Read the model definition and answer for the solid it produces. Units are mm, in the model's axes. Face numbers are marked on the shaded views. A direction names the side the tool comes from. Give positions to 0.01 mm unless a question says otherwise; leave off trailing zeros. Write each loop counter-clockwise with the first axis right and the second up, starting at its lowest first coordinate (ties: lowest second). Pieces come first, ordered by that corner, then holes.
```python
from build123d import *

# Parameters (mm, degrees)
SKETCH1_W           = 28.956
SKETCH1_H           = 8.9916
SKETCH1_R           = 1.6002
BOSS_EXTRUDE1_DEPTH = 3.048
SKETCH2_W           = 7.62
SKETCH2_H           = 1.905
BOSS_EXTRUDE2_DEPTH = 6.35
FILLET1_R           = 0.254
FILLET2_R           = 0.635
CHAMFER1_SIZE       = 0.635


with BuildPart() as part:
    # Sketch1 → Boss-Extrude1 (new body)
    with BuildSketch(Plane(origin=(0, 0, 0), x_dir=(1, 0, 0), z_dir=(0, 1, 0))):
        Rectangle(SKETCH1_W, SKETCH1_H)
        with Locations(Location((8.128, 0, 0), (0, 0, 90))):
            Circle(SKETCH1_R, mode=Mode.SUBTRACT)
        with Locations(Location((-2.032, 0, 0), (0, 0, 90))):
            Circle(SKETCH1_R, mode=Mode.SUBTRACT)
    extrude(amount=BOSS_EXTRUDE1_DEPTH)

    # Sketch2 → Boss-Extrude2 (add)
    with BuildSketch(Plane.XY.offset(4.4958)):
        with Locations((-10.668, -0.9525)):
            Rectangle(SKETCH2_W, SKETCH2_H)
    extrude(amount=-BOSS_EXTRUDE2_DEPTH)

    # Fillet1
    fillet1_edges = [part.edges().sort_by_distance(p)[0] for p in [
        (-10.668, 0, -1.8542),
        (-6.858, 0, 1.3208),
    ]]
    fillet(fillet1_edges, radius=FILLET1_R)

    # Fillet2
    fillet2_edges = [part.edges().sort_by_distance(p)[0] for p in [
        (14.478, 1.524, 4.4958),
        (-14.478, 0.5715, 4.4958),
        (-14.478, 1.524, -4.4958),
        (14.478, 1.524, -4.4958),
    ]]
    fillet(fillet2_edges, radius=FILLET2_R)

    # Chamfer1
    chamfer1_edges = [part.edges().sort_by_distance(p)[0] for p in [
        (0, 3.048, -4.4958),
        (14.478, 3.048, 0),
        (-14.478, 3.048, 0),
        (0, 3.048, 4.4958),
        (-14.292012806, 3.048, -4.309812806),
        (-14.292012806, 3.048, 4.309812806),
        (14.292012806, 3.048, 4.309812806),
        (14.292012806, 3.048, -4.309812806),
    ]]
    chamfer(chamfer1_edges, length=CHAMFER1_SIZE)


solid = part.part
```
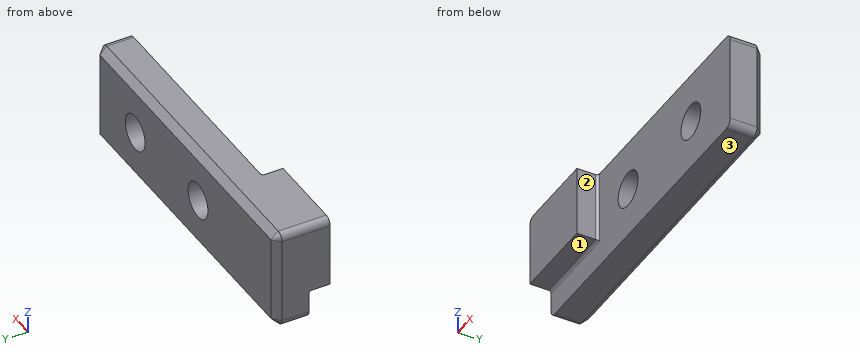
Item 1: Section A-A (z = 0) is taken. Write down the section's boundary in (x, y) (3 decimals).
Result set:
outline: (-14.478, -1.905) - (-6.858, -1.905) - (-6.858, -0.254) arc R0.254 cw to (-6.604, 0) - (-3.632, 0) - (-3.632, 3.048) - (-13.843, 3.048) - (-14.478, 2.413) - close; (-0.432, 0) - (6.528, 0) - (6.528, 3.048) - (-0.432, 3.048) - close; (9.728, 0) - (14.478, 0) - (14.478, 2.413) - (13.843, 3.048) - (9.728, 3.048) - close
Item 2: Find the intervals of material crossed by line 1 along X through (y, z) = (2.2, 0); line 2 along X through (y, z) = (2.55, 0.5); line 3 along X through (y, z) = (-0.4, -1), in increasing order.
Result set:
line 1: x = -14.48 to -3.63, -0.43 to 6.53, 9.73 to 14.48
line 2: x = -14.34 to -3.55, -0.51 to 6.61, 9.65 to 14.34
line 3: x = -14.48 to -6.86
Item 3: Each of these flat-tipped pins is pushed along its axis until it touches: pin 1 Ø3 at (x, z) = (8.128, 0) entering from +Y; pin 2 Ø4 at (x, z) = (-2.032, 0) entering from -Y; pin 3 Ø0.5 at (x, y) = (-11, -1) entering from -Z; pin 4 Ø1.3 at (y, z) = (-1.5, 0) entering from +X. Where does it stop, or does it pass through?
Result set:
pin 1: passes through
pin 2: stops at y = 0
pin 3: stops at z = -1.85
pin 4: stops at x = -6.86
Item 4: Section C-C (z = 2.5) is taken. Write down the section's boundary in (x, y) (3 decimals), and give its area (3 significant figures).
Result set:
outline: (-14.478, -1.905) - (-6.858, -1.905) - (-6.858, -0.254) arc R0.254 cw to (-6.604, 0) - (14.478, 0) - (14.478, 2.413) - (13.843, 3.048) - (-13.843, 3.048) - (-14.478, 2.413) - close
area: 102 mm2
Item 5: Section D-D (y = 1.65) is taken. Write down the section's boundary in (x, z) (3 decimals), and give its area (3 significant figures).
Result set:
outline: (-14.478, -3.861) arc R0.635 ccw to (-13.843, -4.496) - (13.843, -4.496) arc R0.635 ccw to (14.478, -3.861) - (14.478, 3.861) arc R0.635 ccw to (13.843, 4.496) - (-13.843, 4.496) arc R0.635 ccw to (-14.478, 3.861) - close; hole circle Ø3.2 at (-2.032, 0); hole circle Ø3.2 at (8.128, 0)
area: 244 mm2
Item 6: Which of the six approach directions +Z, -Z, +X, -X, +Y, -Y give full straight-line access (tool end or side, diameter ignored) to the marked faces 1, 2 and 3?
Result set:
face 1: -Z, +X, -X, -Y
face 2: +Z, -Z, +X, -Y
face 3: -Z, +X, -X, +Y, -Y
Item 7: Section B-B (x = 10.75) is taken. Write down the section's boundary in (y, z), and give its area (3 significant figures).
Result set:
outline: (0, -4.5) - (2.41, -4.5) - (3.05, -3.86) - (3.05, 3.86) - (2.41, 4.5) - (0, 4.5) - close
area: 27.0 mm2
